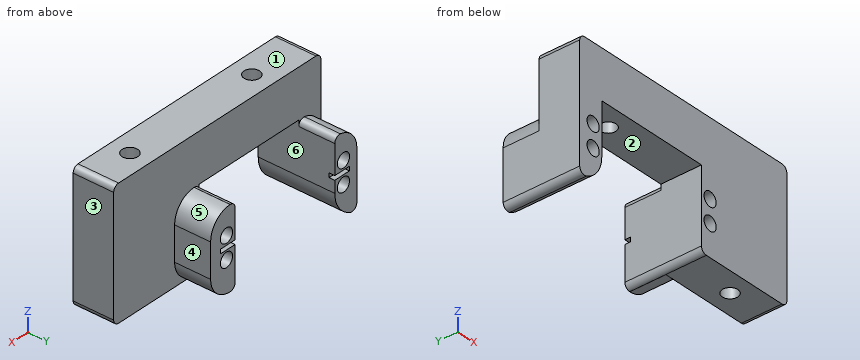
```python
from build123d import *

# Parameters (mm, degrees)
SKETCH1_W           = 85
SKETCH1_H           = 45
BOSS_EXTRUDE1_DEPTH = 27
SKETCH2_R           = 2.5
CUT_EXTRUDE1_DEPTH  = 100.894944817
SKETCH4_W           = 17
SKETCH4_H           = 12.7
CUT_EXTRUDE2_DEPTH  = 100.894944817
SKETCH5_W           = 25
SKETCH5_H           = 12.7
CUT_EXTRUDE3_DEPTH  = 94.477269964
SKETCH6_W           = 40.9
SKETCH6_H           = 28
CUT_EXTRUDE4_DEPTH  = 100.894944817
FILLET1_R           = 10
FILLET2_R           = 8
FILLET4_R           = 2
SKETCH7_R           = 2.75
CUT_EXTRUDE5_DEPTH  = 100.894944817
SKETCH8_W           = 6
SKETCH8_H           = 1.5
CUT_EXTRUDE6_DEPTH  = 2


with BuildPart() as part:
    # Sketch1 → Boss-Extrude1 (new body)
    with BuildSketch(Plane(origin=(0, 0, 0), x_dir=(1, 0, 0), z_dir=(0, 1, 0))):
        with Locations((42.5, 22.5)):
            Rectangle(SKETCH1_W, SKETCH1_H)
    extrude(amount=BOSS_EXTRUDE1_DEPTH)

    # Sketch2 → Cut-Extrude1 (cut, through all)
    with BuildSketch(Plane(origin=(0, 27, 0), x_dir=(1, 0, 0), z_dir=(0, 1, 0))):
        with Locations(Location((5.5, 34, 0), (0, 0, 270))):
            Circle(SKETCH2_R)
        with Locations(Location((53.5, 34, 0), (0, 0, 270))):
            Circle(SKETCH2_R)
        with Locations(Location((53.5, 26.2, 0), (0, 0, 270))):
            Circle(SKETCH2_R)
        with Locations(Location((5.5, 26.2, 0), (0, 0, 270))):
            Circle(SKETCH2_R)
    extrude(amount=-CUT_EXTRUDE1_DEPTH, mode=Mode.SUBTRACT)

    # Sketch4 → Cut-Extrude2 (cut, through all)
    with BuildSketch(Plane.ZY):
        with Locations((-8.5, 20.65)):
            Rectangle(SKETCH4_W, SKETCH4_H)
    extrude(amount=-CUT_EXTRUDE2_DEPTH, mode=Mode.SUBTRACT)

    # Sketch5 → Cut-Extrude3 (cut, through all)
    with BuildSketch(Plane.XY.offset(-17)):
        with Locations((72.5, 20.65)):
            Rectangle(SKETCH5_W, SKETCH5_H)
    extrude(amount=-CUT_EXTRUDE3_DEPTH, mode=Mode.SUBTRACT)

    # Sketch6 → Cut-Extrude4 (cut, through all)
    with BuildSketch(Plane(origin=(0, 27, 0), x_dir=(1, 0, 0), z_dir=(0, 1, 0))):
        with Locations((29.5, 31)):
            Rectangle(SKETCH6_W, SKETCH6_H)
    extrude(amount=-CUT_EXTRUDE4_DEPTH, mode=Mode.SUBTRACT)

    # Fillet1
    # the kernel refuses this fillet: 10 mm, written as the material it takes off along each edge
    with BuildSketch(Plane(origin=(9.05, 51.886931812, -45), x_dir=(-1, 0, 0), z_dir=(0, -1, 0))) as fillet1_piece_1:
        with BuildLine():
            CenterArc((10, -9.954772725), FILLET1_R, 95.451319812, 84.548680188)
            Line((0, -9.954772725), (-0.2, -9.954772725))
            Line((-0.2, -9.954772725), (-0.2, 0))
            Line((-0.2, 0), (0, 0.2))
            ThreePointArc((0, 0.2), (4.525, 0.2), (9.031, 0.199095454))
            Line((9.031, 0.199095454), (9.05, 0))
        make_face()
    extrude(amount=76.773863623, mode=Mode.SUBTRACT)

    # Fillet2
    fillet2_edges = [part.edges().sort_by_distance(p)[0] for p in [
        (0, 20.65, -17),
        (60, 20.65, -45),
        (60, 20.65, -17),
    ]]
    fillet(fillet2_edges, radius=FILLET2_R)

    # Fillet4
    # the kernel refuses this fillet: 2 mm, written as the material it takes off along each edge
    with BuildSketch(Plane(origin=(9.05, 32.797158858, -17), x_dir=(0, 0, -1), z_dir=(0, -1, 0))) as fillet4_piece_1:
        with BuildLine():
            CenterArc((2.075685694, -2), FILLET4_R, 90, 99.110170153)
            Line((0.100914258, -2.316666667), (-0.096562885, -2.348333333))
            ThreePointArc((-0.096562885, -2.348333333), (-0.2, -1.05), (-0.2, 0))
            Line((-0.2, 0), (0, 0.2))
            Line((0, 0.2), (2.075685694, 0.2))
            Line((2.075685694, 0.2), (2.075685694, 0))
        make_face()
    extrude(amount=18.497158858, mode=Mode.SUBTRACT)
    with BuildSketch(Plane(origin=(49.95, 32, -17), x_dir=(0, 0, -1), z_dir=(0, -1, 0))) as fillet4_piece_2:
        with BuildLine():
            CenterArc((FILLET4_R, FILLET4_R), FILLET4_R, 180, 90)
            Line((0, FILLET4_R), (0, 0))
            Line((0, 0), (FILLET4_R, 0))
        make_face()
    extrude(amount=17.7, mode=Mode.SUBTRACT)
    with BuildSketch(Plane(origin=(49.95, 32, -45), x_dir=(0, 0, 1), z_dir=(0, -1, 0))) as fillet4_piece_3:
        with BuildLine():
            CenterArc((FILLET4_R, -FILLET4_R), FILLET4_R, 90, 90)
            Line((0, -FILLET4_R), (0, 0))
            Line((0, 0), (FILLET4_R, 0))
        make_face()
    extrude(amount=37, mode=Mode.SUBTRACT)
    with BuildSketch(Plane(origin=(85, -5, -45), x_dir=(0, 0, 1), z_dir=(0, 1, 0)), Plane(origin=(85, -5, 0), x_dir=(-1, 0, 0), z_dir=(0, 1, 0)), Plane(origin=(0, -5, 0), x_dir=(0, 0, -1), z_dir=(0, 1, 0))) as fillet4_piece_4:
        with BuildLine():
            CenterArc((FILLET4_R, -FILLET4_R), FILLET4_R, 90, 90)
            Line((0, -FILLET4_R), (0, 0))
            Line((0, 0), (FILLET4_R, 0))
        make_face()
    extrude(amount=24.3, mode=Mode.SUBTRACT)
    with BuildSketch(Plane(origin=(0, -7.039544043, -45), x_dir=(0.972186544788057, 0, 0.23420786095487744), z_dir=(0, 1, 0))) as fillet4_piece_5:
        with BuildLine():
            CenterArc((2.534235855, -1.980078713), FILLET4_R, 81.906386313, 111.638547186)
            Line((0.589862766, -2.448494435), (0, 0))
            ThreePointArc((0, 0), (1.407908809, 0.099606433), (2.815817617, 0))
        make_face()
    extrude(amount=41.079088086, mode=Mode.SUBTRACT)

    # Sketch7 → Cut-Extrude5 (cut, through all)
    with BuildSketch(Plane.XY):
        with Locations((70, 7.15)):
            Circle(SKETCH7_R)
        with Locations((20, 7.15)):
            Circle(SKETCH7_R)
    extrude(amount=-CUT_EXTRUDE5_DEPTH, mode=Mode.SUBTRACT)

    # Sketch8 → Cut-Extrude6 (cut)
    with BuildSketch(Plane(origin=(0, 27, 0), x_dir=(1, 0, 0), z_dir=(0, 1, 0))):
        with Locations((6.05, 30.1)):
            Rectangle(SKETCH8_W, SKETCH8_H)
        with Locations((52.95, 30.1)):
            Rectangle(SKETCH8_W, SKETCH8_H)
    extrude(amount=-CUT_EXTRUDE6_DEPTH, mode=Mode.SUBTRACT)


solid = part.part
```
Geometry check sheet. Reference: the model listing, model coordinates, mm. Face numbers are marked on the shaded views. A direction names the side the tool comes from. Round coordinates to 2 decimals unless told otherwise and drop trailing zeros. Write each loop counter-clockwise with the first axis right and the second up, starting at its lowest first coordinate (ties: lowest second). Pieces come first, ordered by that corner, then holes. Notation, with made-up numbers: (14.5, 5.25) - (32.5, 5.25) arc R24 ccw to (32.5, 31.25) - close; hole circle Ø6 at (48.25, 76.25). An arc over 180 degrees is marked (long way). Write each question's results on one line, items separated by ' | '.
(1) Sectioned sample at D-D, the plane x = 20. Enter the section's corners in (y, z).
Computed:
outline: (0, -17) - (4.4, -17) - (4.4, 0) - (0, 0) - close; (9.9, -17) - (14.3, -17) - (14.3, 0) - (9.9, 0) - close
(2) Sectioned sample at B-B, the plane z = -26.2. Enter the section's corners in (x, y), plus the area to 3 significant figures.
Computed:
outline: (0, 0) - (3, 0) - (3, 27) - (0, 27) - close; (8, 0) - (9.05, 0) - (9.05, 27) - (8, 27) - close; (49.95, 0) - (51, 0) - (51, 27) - (49.95, 27) - close; (56, 0) - (85, 0) - (85, 14.3) - (60, 14.3) - (60, 27) - (56, 27) - close; hole circle Ø5.5 at (70, 7.15) | area: 579 mm^2
(3) Depth check by flat-ended pin: pin 1 Ø3 at (x, z) = (64.5, -27) entering from +Y; pin 2 Ø3.5 at (x, y) = (70, 7.15) entering from -Z; pin 3 Ø1 at (x, y) = (53, 25.5) entering from -Z; pin 4 Ø1.2 at (y, z) = (26, -30) entering from +X. Enter the tip coordinate at first touch or a pass-through.
Computed:
pin 1: stops at y = 14.3 | pin 2: passes through | pin 3: stops at z = -44.98 | pin 4: stops at x = 60
(4) Sectioned sample at A-A, the plane y = 7.15. Enter the section's corners in (x, z).
Computed:
outline: (0, -42.48) arc R2 ccw to (2.74, -44.34) arc R10 ccw to (9.05, -35.05) - (9.05, -17) - (17.25, -17) - (17.25, 0) - (2, 0) arc R2 ccw to (0, -2) - close; (22.75, -17) - (49.95, -17) - (49.95, -43) arc R2 ccw to (51.95, -45) - (67.25, -45) - (67.25, 0) - (22.75, 0) - close; (72.75, -45) - (83, -45) arc R2 ccw to (85, -43) - (85, -2) arc R2 ccw to (83, 0) - (72.75, 0) - close; hole circle Ø5 at (5.5, -34); hole circle Ø5 at (5.5, -26.2); hole circle Ø5 at (53.5, -34); hole circle Ø5 at (53.5, -26.2)
(5) Set-up check for the marked faces 4, 5 and 6: record each of +Z, -Z, +X, -X, +Y, -Y from which the full face is reachable in a straight line by a thin tool's end or side.
Computed:
face 4: +Z, -Z, +X, +Y | face 5: +Z, +X, +Y | face 6: -Z, +Y, -Y
(6) Thickness scan on probe 1 along X at (y, z) = (17, -34); probe 2 along Y at (x, z) = (70, -23.5); probe 3 along X at (y, z) = (1.5, -21.5). Record the ranges inside material, lowest first. Write a range as from..to.
Computed:
probe 1: x = 0..3, 8..9.05, 49.95..51, 56..60 | probe 2: y = 0..4.4, 9.9..14.3 | probe 3: x = 0..9.05, 49.95..85
(7) Sectioned sample at C-C, the plane y = 18.75. Enter the section's corners in (x, z), plus the area to 3 significant figures.
Computed:
outline: (0, -42.48) arc R2 ccw to (2.74, -44.34) arc R10 ccw to (9.05, -35.05) - (9.05, -19.08) arc R2 ccw to (6.73, -17.1) arc R8 ccw to (0, -25) - close; (49.95, -43) arc R2 ccw to (51.95, -45) - (52, -45) arc R8 ccw to (60, -37) - (60, -25) arc R8 ccw to (52, -17) - (51.95, -17) arc R2 ccw to (49.95, -19) - close; hole circle Ø5 at (5.5, -34); hole circle Ø5 at (5.5, -26.2); hole circle Ø5 at (53.5, -34); hole circle Ø5 at (53.5, -26.2) | area: 390 mm^2
(8) Draft check along X on the marked faces 1, 2 and 3. Enter one of: pulls with the +X half, pulls with the -X half, needs draft (parallel to the pull), parting line crosses it, or undercut.
Computed:
face 1: needs draft | face 2: undercut | face 3: pulls with the +X half
